```python
from build123d import *

# Parameters (mm, degrees)
SKETCH1_R           = 6
BOSS_EXTRUDE1_DEPTH = 14
SKETCH2_R           = 5.6261
CUT_EXTRUDE1_DEPTH  = 0.7366


with BuildPart() as part:
    # Sketch1 → Boss-Extrude1 (new body)
    with BuildSketch(Plane(origin=(0, 0, 0), x_dir=(1, 0, 0), z_dir=(0, 1, 0))):
        Circle(SKETCH1_R)
    extrude(amount=BOSS_EXTRUDE1_DEPTH)

    # Sketch2 → Cut-Extrude1 (cut)
    with BuildSketch(Plane(origin=(0, 2.57, 0), x_dir=(1, 0, 0), z_dir=(0, 1, 0))):
        Polygon((-7.915464339, 6.772300258), (-7.748596028, -7.998854616), (10.395730316, -7.998854616), (9.153265383, 7.840750397), align=None)
        Circle(SKETCH2_R, mode=Mode.SUBTRACT)
    extrude(amount=-CUT_EXTRUDE1_DEPTH, mode=Mode.SUBTRACT)


solid = part.part
```
The model under review builds one solid part; all positions refer to its coordinate system, in mm. Round coordinates to 2 decimals unless told otherwise and drop trailing zeros. Write each loop counter-clockwise with the first axis right and the second up, starting at its lowest first coordinate (ties: lowest second). Pieces come first, ordered by that corner, then holes.
(1) We need section A-A on x = 3.75. Give the boundary of the cut face in (y, z).
(2) We need section B-B on y = 13.25. Give the boundary of the cut face in (x, z).
(3) Insertion check: pin 1 (5 mm diameter, centred on y = 9, z = -4.5, fed in from +X); pin 2 (1 mm diameter, centred on x = 3, y = 10, fed in from +Z). Each pin has a flat end and moves straight along its axis. Give the tip position at first contact, or say it passes through.
(4) Wall thickness on L1, parallel to X at y = 10.75, z = 5.25; L2, parallel to Z at x = 3.75, y = 4.75; L3, parallel to X at y = 5.25, z = 0.5: over which ranges is each line inside the solid? List them lowest first.
(5) We need section C-C on z = -1.5. Give the boundary of the cut face in (x, y).
(6) Mouldability with a two-part tool opening along Y and no side actions: class faces 1 (the flat face through (0, 0, 0)), 2 (the cylindrical face through (-6, 8, 0)), 3 (the flat face through (0, 14, 0)), 4 (the cylindrical face through (-0.73, 2.21, -5.58)) as +Y half, -Y half, draft (parallel to the pull), parting line (faces both ways), or undercut.
Findings below:
1. outline: (0, -4.68) - (1.83, -4.68) - (1.83, -4.19) - (2.57, -4.19) - (2.57, -4.68) - (14, -4.68) - (14, 4.68) - (2.57, 4.68) - (2.57, 4.19) - (1.83, 4.19) - (1.83, 4.68) - (0, 4.68) - close
2. outline: circle Ø12 at (0, 0)
3. pin 1: stops at x = 5.66
3. pin 2: stops at z = 5.45
4. L1: x = -2.9 to 2.9
4. L2: z = -4.68 to 4.68
4. L3: x = -5.98 to 5.98
5. outline: (-5.81, 0) - (5.81, 0) - (5.81, 1.83) - (5.42, 1.83) - (5.42, 2.57) - (5.81, 2.57) - (5.81, 14) - (-5.81, 14) - (-5.81, 2.57) - (-5.42, 2.57) - (-5.42, 1.83) - (-5.81, 1.83) - close
6. face 1: -Y half
6. face 2: draft
6. face 3: +Y half
6. face 4: undercut
